The drawing under review shows one solid part. Ordinate dimensions are in mm from its lowest x, y, z. A direction names the side the tool comes from. Give positions to 0.01 mm unless a question says otherwise; leave off trailing zeros. Write each loop counter-clockwise with the first axis right and the second up, starting at its lowest first coordinate (ties: lowest second). Pieces come first, ordered by that corner, then holes. Notation, with made-up numbers: M -22,-15 L 24,-15 A23 ccw 24,-4 Z; hole C 10,78 d9. An arc over 180 degrees is marked long. Use one line per item in the form item = value. Start each with the question number.
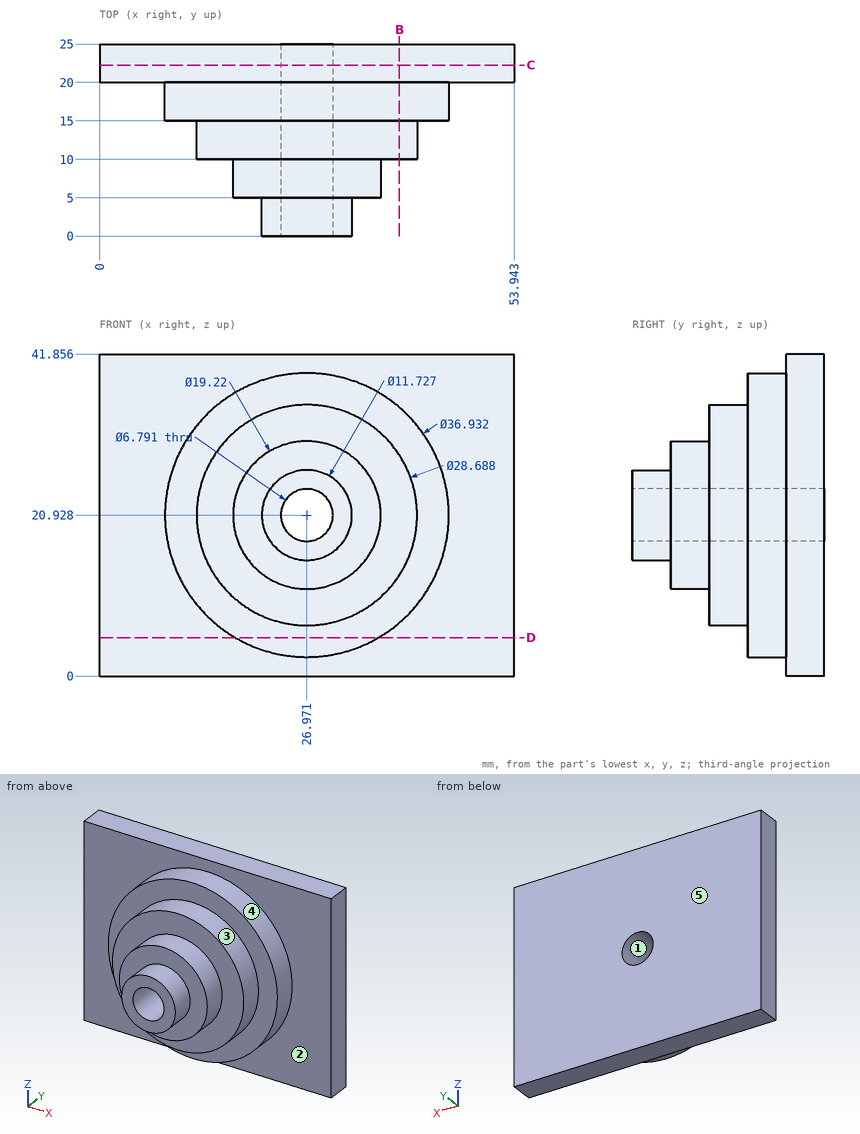
1. We need section D-D (z = 5). State the section outline as (x, y) points (1 decimal).
2. Clearance check with flat-ended pins moving along their axes: pin 1 Ø2 at (y, z) = (12, 21.5) entering from +X (1 decimal); pin 2 Ø4 at (x, y) = (43, 15.5) entering from +Z (1 decimal); pin 3 Ø6 at (x, y) = (23, 3) entering from -Z (1 decimal). State where each tip first meets the part, or that it passes through.
3. We need section C-C (y = 22.25). State the section outline as (x, z) points (1 decimal).
4. For the marked faces 4 and 5, list the 3-axis set-ups (+Z, -Z, +X, -X, +Y, -Y) from which the entire face can be reached by the end or side of a thin tool; tool diameter is ignored.
5. To check wall thickness, follow L1, parallel to Y at x = 32, z = 7; L2, parallel to Y at x = 11.5, z = 40; L3, parallel to X at y = 22, z = 22. State the ranges of each line that lie inside material, in increasing order.
6. We need section B-B (x = 39). State the section outline as (y, z) points (1 decimal).
7. Draft analysis for pull direction X (two halves, no side actions). For the marked faces 1, 2 and 3, state which applies: pulls with the +X half, pulls with the -X half, needs draft (parallel to the pull), parting line crosses it, or undercut.
Answer block:
q1.outline = M 0,20 L 17.6,20 L 17.6,15 L 36.3,15 L 36.3,20 L 53.9,20 L 53.9,25 L 0,25 Z
q2.pin_1 = 41.3
q2.pin_2 = 32.9
q2.pin_3 = 11.5
q3.outline = M 0,0 L 53.9,0 L 53.9,41.9 L 0,41.9 Z; hole C 27,20.9 d6.8
q4.face_4 = -Y
q4.face_5 = +Z, -Z, +X, -X, +Y
q5.L1 = 15 to 25
q5.L2 = 20 to 25
q5.L3 = 0 to 23.75, 30.19 to 53.94
q6.outline = M 10,13.1 L 15,13.1 L 15,6.9 L 20,6.9 L 20,0 L 25,0 L 25,41.9 L 20,41.9 L 20,34.9 L 15,34.9 L 15,28.7 L 10,28.7 Z
q7.face_1 = undercut
q7.face_2 = needs draft
q7.face_3 = parting line crosses it
